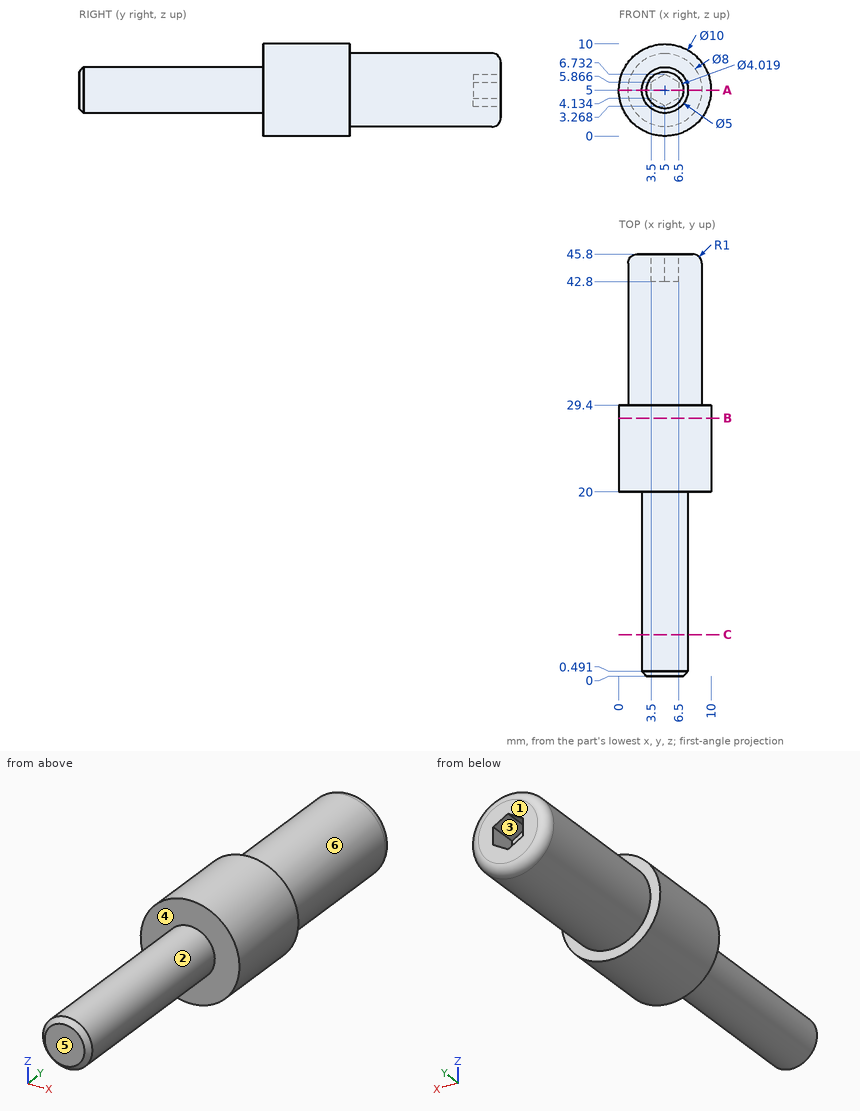
Answer from the drawing. Dimensions are ordinates in mm from the lowest x, y and z of the part. A direction names the side the tool comes from. Give positions to 0.01 mm unless a question says otherwise; leave off trailing zeros. Order: outer loops, then holes, each group sorted by start corner. A loop starts at its lowest first (then second) coordinate and runs counter-clockwise, first axis right, second up. Notation, with made-up numbers: (78, 48.5) - (121, 48.5) arc R29 ccw to (121, 72.5) - close; hole circle Ø8 at (70.5, -5). An arc over 180 degrees is marked (long way). One line per item, written item: value. Start each with the question number.
1) Find the intervals of material crossed by L1, parallel to X at y = 34, z = 5; L2, parallel to Y at x = 4, z = 1; L3, parallel to Y at x = 4, z = 4.25, in increasing order.
2) Given pin 1 Ø4 at (y, z) = (8, 5) entering from +X; pin 2 Ø3 at (x, y) = (8.5, 20.5) entering from +Z; pin 3 Ø1.9 at (y, z) = (43.5, 4.5) entering from +X, each flat-ended and moving along its own axis, determine where each tip first touches the part or whether it passes through.
3) The mould has two halves that part along Z. Classify the marked faces 1, 2 and 3: released by +Z, released by -Z, zero draft, split by the parting line, or undercut.
4) A cutting plane is placed at B-B on y = 28. Give the vertices of the cut face in (x, z).
5) A cutting plane is placed at A-A on z = 5. Give the vertices of the cut face in (x, y).
6) A tool of negligible diameter and unlimited length cuts with its end or side. For the marked faces 4, 5 and 6, from which of +Z, -Z, +X, -X, +Y, -Y can it reach the whole face along a straight path? Write none if from no direction.
7) A cutting plane is placed at C-C on y = 4.5. Give the vertices of the cut face in (x, z).
Answer sheet:
1. L1: x = 1 to 9
1. L2: y = 20 to 29.4
1. L3: y = 0 to 42.8
2. pin 1: stops at x = 7.5
2. pin 2: stops at z = 9.58
2. pin 3: stops at x = 9
3. face 1: zero draft
3. face 2: split by the parting line
3. face 3: undercut
4. outline: circle Ø10 at (5, 5)
5. outline: (0, 20) - (2.5, 20) - (2.5, 0.49) - (2.99, 0) - (7.01, 0) - (7.5, 0.49) - (7.5, 20) - (10, 20) - (10, 29.4) - (9, 29.4) - (9, 44.8) arc R1 ccw to (8, 45.8) - (6.5, 45.8) - (6.5, 42.8) - (3.5, 42.8) - (3.5, 45.8) - (2, 45.8) arc R1 ccw to (1, 44.8) - (1, 29.4) - (0, 29.4) - close
6. face 4: -Y
6. face 5: +Z, -Z, +X, -X, -Y
6. face 6: +Y
7. outline: circle Ø5 at (5, 5)
